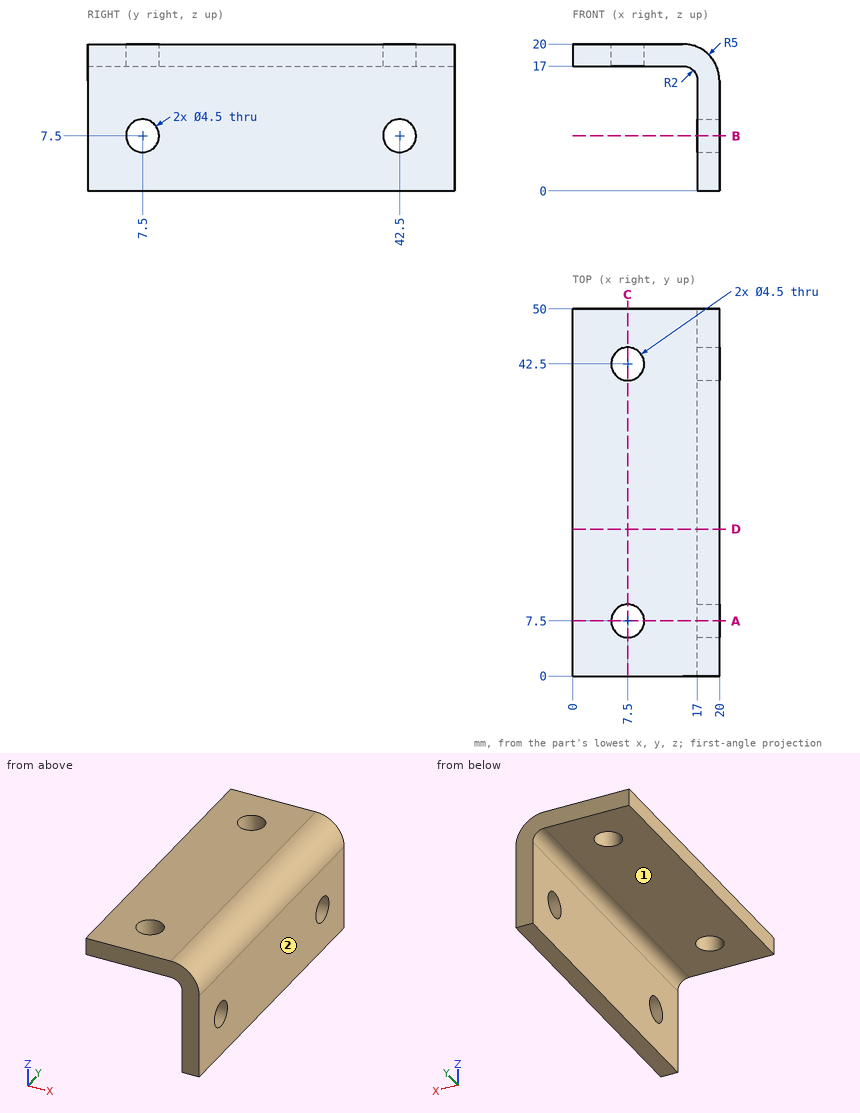
Geometry check sheet. Reference: drawing and pictorial views, mm from the part's lowest x, y, z. A direction names the side the tool comes from. Round coordinates to 2 decimals unless told otherwise and drop trailing zeros. Loops run counter-clockwise (first coordinate to the right, second up) from the corner with the lowest first, then second, coordinate; pieces in that order, holes last. Notation, with made-up numbers: (75.5, -18) -> (132.5, -18) arc R20 ccw to (132.5, -5) -> close; hole circle Ø6 at (-21, 23.25). An arc over 180 degrees is marked (long way). Answer as a JSON object with one key per item and string values.
Q1. Section check D-D (y = 20). Record the boundary of the cut face in (x, z).
Data:
{"outline": "(0, 17) -> (15, 17) arc R2 cw to (17, 15) -> (17, 0) -> (20, 0) -> (20, 15) arc R5 ccw to (15, 20) -> (0, 20) -> close"}
Q2. Section check C-C (x = 7.5). Record the boundary of the cut face in (y, z).
Data:
{"outline": "(0, 17) -> (5.25, 17) -> (5.25, 20) -> (0, 20) -> close; (9.75, 17) -> (40.25, 17) -> (40.25, 20) -> (9.75, 20) -> close; (44.75, 17) -> (50, 17) -> (50, 20) -> (44.75, 20) -> close"}
Q3. Section check B-B (z = 7.5). Record the boundary of the cut face in (x, y), then the cut area to 3 significant figures.
Data:
{"outline": "(17, 0) -> (20, 0) -> (20, 5.25) -> (17, 5.25) -> close; (17, 9.75) -> (20, 9.75) -> (20, 40.25) -> (17, 40.25) -> close; (17, 44.75) -> (20, 44.75) -> (20, 50) -> (17, 50) -> close", "area": "123 mm2"}
Q4. Scan lines: line 1 (Y direction, x = 7.5, z = 19.3); line 2 (X direction, y = 45.5, z = 6.25); line 3 (X direction, y = 42.5, z = 19.45). Record each from-to range of solid material in increasing order. Write a range as from..to.
Data:
{"line 1": "y = 0..5.25, 9.75..40.25, 44.75..50", "line 2": "x = 17..20", "line 3": "x = 0..5.25, 9.75..17.28"}
Q5. Go/stop test with flat-tipped pins: P1, Ø7.5, axis at x = 4.5, y = 31.5, coming from the -Z side; P2, Ø3.5, axis at y = 42.5, z = 7.5, coming from the +X side; P3, Ø4, axis at y = 36, z = 3, coming from the -X side. Record where each tip stops, or that it passes through.
Data:
{"P1": "stops at z = 17", "P2": "passes through", "P3": "stops at x = 17"}
Q6. Access from +Z, -Z, +X, -X, +Y, -Y to the whole of each face (thin tool, end or side, straight path). Record for the marked faces 1 and 2.
Data:
{"face 1": "-Z, -X, +Y, -Y", "face 2": "+Z, -Z, +X, +Y, -Y"}
Q7. Section check A-A (y = 7.5). Record the boundary of the cut face in (x, z), then the cut area to 3 significant figures.
Data:
{"outline": "(0, 17) -> (5.25, 17) -> (5.25, 20) -> (0, 20) -> close; (9.75, 17) -> (15, 17) arc R2 cw to (17, 15) -> (17, 9.75) -> (20, 9.75) -> (20, 15) arc R5 ccw to (15, 20) -> (9.75, 20) -> close; (17, 0) -> (20, 0) -> (20, 5.25) -> (17, 5.25) -> close", "area": "79.5 mm2"}
